```python
from build123d import *

# Parameters (mm, degrees)
BOSS_EXTRUDE1_DEPTH = 70
SKETCH2_R           = 40
CUT_EXTRUDE1_DEPTH  = 10
SKETCH3_R           = 23
CUT_EXTRUDE2_DEPTH  = 66
SKETCH4_W           = 30
SKETCH4_H           = 15
SKETCH4_H_2         = 20
CUT_EXTRUDE3_DEPTH  = 10


with BuildPart() as part:
    # Sketch1 → Boss-Extrude1 (new body)
    with BuildSketch(Plane.XY):
        with BuildLine():
            Line((-60.063092464, -25.71543861), (-60.063092464, -45.71543861))
            Line((-60.063092464, -45.71543861), (-30.063092464, -45.71543861))
            Line((-30.063092464, -45.71543861), (-30.063092464, -30.71543861))
            Line((-30.063092464, -30.71543861), (29.936907536, -30.71543861))
            Line((29.936907536, -30.71543861), (29.936907536, -45.71543861))
            Line((29.936907536, -45.71543861), (59.936907536, -45.71543861))
            Line((59.936907536, -45.71543861), (59.936907536, -25.71543861))
            ThreePointArc((59.936907536, -25.71543861), (44.936907536, -10.71543861), (59.936907536, 4.28456139))
            Line((59.936907536, 4.28456139), (59.936907536, 24.28456139))
            Line((59.936907536, 24.28456139), (29.936907536, 24.28456139))
            Line((29.936907536, 24.28456139), (29.936907536, 14.28456139))
            Line((29.936907536, 14.28456139), (12.436907536, 14.28456139))
            Line((12.436907536, 14.28456139), (12.436907536, -5.71543861))
            Line((12.436907536, -5.71543861), (-12.563092464, -5.71543861))
            Line((-12.563092464, -5.71543861), (-12.563092464, 14.28456139))
            Line((-12.563092464, 14.28456139), (-30.063092464, 14.28456139))
            Line((-30.063092464, 14.28456139), (-30.063092464, 24.28456139))
            Line((-30.063092464, 24.28456139), (-60.063092464, 24.28456139))
            Line((-60.063092464, 24.28456139), (-60.063092464, 4.28456139))
            ThreePointArc((-60.063092464, 4.28456139), (-45.063092464, -10.71543861), (-60.063092464, -25.71543861))
        make_face()
    extrude(amount=BOSS_EXTRUDE1_DEPTH)

    # Sketch2 → Cut-Extrude1 (cut)
    with BuildSketch(Plane(origin=(0, 24.28456139, 0), x_dir=(1, 0, 0), z_dir=(0, 1, 0))):
        with Locations((-0.063092464, -35)):
            Circle(SKETCH2_R)
    extrude(amount=-CUT_EXTRUDE1_DEPTH, mode=Mode.SUBTRACT)

    # Sketch3 → Cut-Extrude2 (cut)
    with BuildSketch(Plane(origin=(0, 14.28456139, 0), x_dir=(1, 0, 0), z_dir=(0, 1, 0))):
        with Locations(Location((-0.063092464, -35, 0), (0, 0, 270))):
            Circle(SKETCH3_R)
    extrude(amount=-CUT_EXTRUDE2_DEPTH, mode=Mode.SUBTRACT)

    # Sketch4 → Cut-Extrude3 (cut)
    with BuildSketch(Plane.ZY.offset(60.063092464)):
        with Locations((35, -18.21543861)):
            Rectangle(SKETCH4_W, SKETCH4_H)
        with Locations((35, -35.71543861)):
            Rectangle(SKETCH4_W, SKETCH4_H_2)
    cut_extrude3 = extrude(amount=-CUT_EXTRUDE3_DEPTH, mode=Mode.SUBTRACT)

    # Mirror1: Cut-Extrude3 across plane
    add(cut_extrude3.mirror(Plane.ZY.offset(0.063092464)), mode=Mode.SUBTRACT)


solid = part.part
```
Here's how the part is built. I have some questions about the finished solid (model axes, mm). A direction names the side the tool comes from. Coordinates: 2 decimals unless noted, no trailing zeros. Order: outer loops, then holes, each group sorted by start corner. A loop starts at its lowest first (then second) coordinate and runs counter-clockwise, first axis right, second up. Notation, with made-up numbers: M 62.25,-7.5 L 75.25,-7.5 A16 ccw 75.25,20.5 Z; hole C -12,-14 d4. An arc over 180 degrees is marked long. Answer as a JSON object with one key per item and string values. Group by question number.
(1) Suppose I cut it at D-D, the plane y = 18.5. Please give me the cut outline in (x, z), then the cut area to 3 significant figures.
(2) Which directions (+Z, -Z, +X, -X, +Y, -Y) give clear straight access to the entire face, cutting with the end or side of a thin tool? Please do faces 4 (the face through (-50.063, -34, 35)), 5 (the face through (-30.063, -38, 35)), 6 (the face through (-12.563, 4, 62)), 7 (the face through (39.935, 19.355, 35.405)).
(3) Suppose I cut it at B-B, the plane y = -38. Please give me the cut outline in (x, z).
(4) Suppose I cut it at C-C, the plane x = 3. Please give me the cut outline in (y, z).
(5) If we mould it in two halves opening along Z, with no side actions, what happens to faces 1 (the face through (55, -34, 20)), 2 (the face through (29.937, 19, 66)), 3 (the face through (-1, -10, 70))? For each: released by +Z, released by -Z, zero draft, split by the parting line, or undercut.
(6) Suppose I cut it at A-A, the plane z = 35. Please give me the cut outline in (x, y).
(7) I need wall thicknesses on probe 1 along X at (y, z) = (-37.5, 44); probe 2 along Y at (x, z) = (25, 57); probe 3 along Z at (x, y) = (50, -32). Which ranges of each line are inside material? Lowest first, please.
(8) For pin 1 (1.5 mm diameter, centred on y = -8.5, z = 7, fed in from +X); pin 2 (17.5 mm diameter, centred on x = -1.5, z = 60.5, fed in from +Y); pin 3 (1.5 mm diameter, centred on y = -23.5, z = 33, fed in from -X), each with a flat end and sliding along its axis, tell me the tip position at first contact or that it passes through.
Values found:
{
 "1": {"outline": "M -60.06,0 L -30.06,0 L -30.06,8.54 A40 cw -30.06,61.46 L -30.06,70 L -60.06,70 Z; M 29.94,0 L 59.94,0 L 59.94,70 L 29.94,70 L 29.94,61.46 A40 cw 29.94,8.54 Z", "area": "3,470 mm^2"},
 "2": {"face 4": "-X, -Y", "face 5": "+Z, -Z, -Y", "face 6": "+Z, -Z, +Y", "face 7": "+Y"},
 "3": {"outline": "M -60.06,0 L -30.06,0 L -30.06,70 L -60.06,70 L -60.06,50 L -50.06,50 L -50.06,20 L -60.06,20 Z; M 29.94,0 L 59.94,0 L 59.94,20 L 49.94,20 L 49.94,50 L 59.94,50 L 59.94,70 L 29.94,70 Z"},
 "4": {"outline": "M -30.72,0 L -5.72,0 L -5.72,12.2 L -30.72,12.2 Z; M -30.72,57.8 L -5.72,57.8 L -5.72,70 L -30.72,70 Z"},
 "5": {"face 1": "undercut", "face 2": "zero draft", "face 3": "released by +Z"},
 "6": {"outline": "M -60.06,4.28 A15 cw -50.06,-21.9 L -50.06,-45.72 L -30.06,-45.72 L -30.06,-30.72 L -23.06,-30.72 L -23.06,14.28 L -40.06,14.28 L -40.06,24.28 L -60.06,24.28 Z; M 22.94,-30.72 L 29.94,-30.72 L 29.94,-45.72 L 49.94,-45.72 L 49.94,-21.9 A15 cw 59.94,4.28 L 59.94,24.28 L 39.94,24.28 L 39.94,14.28 L 22.94,14.28 Z"},
 "7": {"probe 1": "x = -50.06 to -30.06, 29.94 to 49.94", "probe 2": "y = -30.72 to 14.28", "probe 3": "z = 0 to 20, 50 to 70"},
 "8": {"pin 1": "stops at x = 45.23", "pin 2": "stops at y = -5.72", "pin 3": "stops at x = -50.06"}
}
